Source: CAD feature listing. Evaluate the final solid. Frame: model axes, mm. Coordinates: 2 decimals unless noted, no trailing zeros. Order: outer loops, then holes, each group sorted by start corner. A loop starts at its lowest first (then second) coordinate and runs counter-clockwise, first axis right, second up.
Item 1: Section B-B on y = 1.1. State how many separate pieces and enclosed holes the cut face has, then the cut area to 3 significant figures.
Item 2: Ray query, line 1 (Z direction, x = 142, y = 0.1); line 2 (Z direction, x = 10, y = -0.9); line 3 (Z direction, x = 124, y = 0.45). Return the intervals inside material, ascending.
Item 3: Section A-A on x = 61.5. Return the cut outline in (y, z).
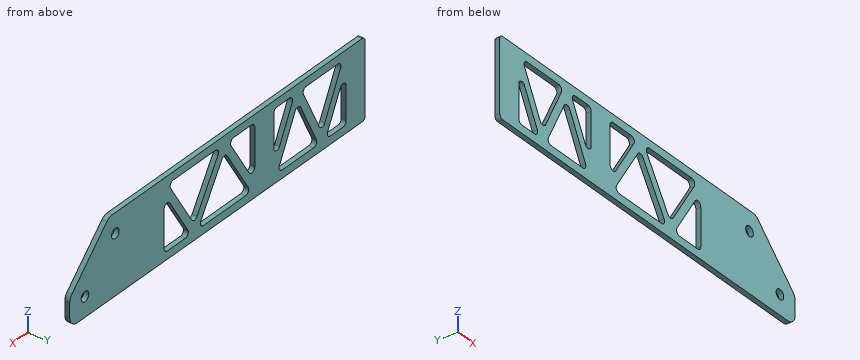
from build123d import *

# Parameters (mm, degrees)
SKETCH1_R           = 3.175
BOSS_EXTRUDE1_DEPTH = 1.5875
FILLET1_R           = 2.54
FILLET2_R           = 6.35


with BuildPart() as part:
    # Sketch1 → Boss-Extrude1 (new body, symmetric)
    with BuildSketch(Plane(origin=(0, 0, 0), x_dir=(1, 0, 0), z_dir=(0, 1, 0))):
        Polygon((121.465512242, -25.4), (154.305, 7.439487758), (154.305, 25.4), (-92.075, 25.4), (-92.075, -25.4), align=None)
        Polygon((-38.817248104, -20.32), (-73.366085229, -20.32), (-56.091666667, 14.592509095), align=None, mode=Mode.SUBTRACT)
        Polygon((-15.875, 14.592509095), (-15.875, -20.32), (-33.149418563, -20.32), align=None, mode=Mode.SUBTRACT)
        Polygon((22.200034711, -20.32), (0, -20.32), (0, 15.498543399), align=None, mode=Mode.SUBTRACT)
        with Locations((116.205, -12.7)):
            Circle(SKETCH1_R, mode=Mode.SUBTRACT)
        Polygon((72.576701378, -20.32), (28.176631956, -20.32), (50.376666667, 15.498543399), align=None, mode=Mode.SUBTRACT)
        Polygon((53.364965289, 20.32), (75.565, 20.32), (75.565, -15.498543399), align=None, mode=Mode.SUBTRACT)
        Polygon((-76.2, -14.592509095), (-76.2, 20.32), (-58.925581437, 20.32), align=None, mode=Mode.SUBTRACT)
        Polygon((-53.257751896, 20.32), (-18.708914771, 20.32), (-35.983333333, -14.592509095), align=None, mode=Mode.SUBTRACT)
        Polygon((2.988298622, 20.32), (47.388368044, 20.32), (25.188333333, -15.498543399), align=None, mode=Mode.SUBTRACT)
        with Locations((141.605, 12.7)):
            Circle(SKETCH1_R, mode=Mode.SUBTRACT)
    extrude(amount=BOSS_EXTRUDE1_DEPTH, both=True)

    # Fillet1
    fillet1_edges = [part.edges().sort_by_distance(p)[0] for p in [
        (-76.2, 0, -20.32),
        (-76.2, 0, 14.592509095),
        (-58.925581437, 0, -20.32),
        (2.988298622, 0, -20.32),
        (25.188333333, 0, 15.498543399),
        (47.388368044, 0, -20.32),
        (0, 0, -15.498543399),
        (0, 0, 20.32),
        (22.200034711, 0, 20.32),
        (72.576701378, 0, 20.32),
        (50.376666667, 0, -15.498543399),
        (28.176631956, 0, 20.32),
        (75.565, 0, 15.498543399),
        (75.565, 0, -20.32),
        (53.364965289, 0, -20.32),
        (-15.875, 0, 20.32),
        (-15.875, 0, -14.592509095),
        (-33.149418563, 0, 20.32),
        (-35.983333333, 0, 14.592509095),
        (-18.708914771, 0, -20.32),
        (-53.257751896, 0, -20.32),
        (-92.075, 0, 25.4),
        (-92.075, 0, -25.4),
        (-38.817248104, 0, 20.32),
        (-56.091666667, 0, -14.592509095),
        (-73.366085229, 0, 20.32),
    ]]
    fillet(fillet1_edges, radius=FILLET1_R)

    # Fillet2
    fillet2_edges = [part.edges().sort_by_distance(p)[0] for p in [
        (154.305, 0, -25.4),
        (154.305, 0, -7.439487758),
        (121.465512242, 0, 25.4),
    ]]
    fillet(fillet2_edges, radius=FILLET2_R)


solid = part.part
Answer list:
1. separate pieces: 1
1. enclosed holes: 10
1. area: 7,850 mm2
2. line 1: z = -25.4 to -15.85, -9.55 to 4.87
2. line 2: z = -25.4 to -20.32, -9.01 to 0.64, 20.32 to 25.4
2. line 3: z = -25.4 to 22.87
3. outline: (-1.59, -25.4) - (1.59, -25.4) - (1.59, -20.32) - (-1.59, -20.32) - close; (-1.59, -7.19) - (1.59, -7.19) - (1.59, 2.45) - (-1.59, 2.45) - close; (-1.59, 20.32) - (1.59, 20.32) - (1.59, 25.4) - (-1.59, 25.4) - close
